Geometry: final body of the model. Coordinates: model frame, mm. A direction names the side the tool comes from. Round coordinates to 2 decimals unless told otherwise and drop trailing zeros. Loops run counter-clockwise (first coordinate to the right, second up) from the corner with the lowest first, then second, coordinate; pieces in that order, holes last. Notation, with made-up numbers: (12.25, 12.25) - (62.25, 12.25) arc R19 cw to (62.25, 25.25) - close; hole circle Ø6 at (73, 14.25). An arc over 180 degrees is marked (long way). Write item = value, one per line. Start each with the question number.
Item 1: Section A-A (y = 33). Return loops of the section in (x, z) (3 decimals).
Item 2: Line query: line 1 (X direction, y = 39, z = 0); line 2 (Y direction, x = -76, z = 5); line 3 (X direction, y = 25, z = 0). Output: solid intervals per line, ascending. Write a range as from..to.
Item 3: First-contact query: pin 1 (8.5 mm diameter, centred on x = 16, y = 30.5, fed in from -Z); pin 2 (4 mm diameter, centred on y = 8, z = -17.5, fed in from -X); pin 3 (10 mm diameter, centred on x = -48.5, y = 12, fed in from +Z); pin 4 (9 mm diameter, centred on x = 0, z = -45, fed in from +Y). Flat tips, straight axial feed; report the tip coordinate or a pass-through.
Item 4: Section C-C (x = 0). Count the separate pieces of the cut face and the enclosed holes in it, plus the area to 4 significant figures.
Item 5: Section D-D (y = 48.5). Return loops of the section in (x, z) (3 decimals), plus the area to 3 significant figures.
Item 6: Section B-B (z = 0). Return loops of the section in (x, y).
Item 7: Access query for faces 4 (the flat face through (0, 37.5, 15)), 5 (the flat face through (67, 15, -1)), 6 (the flat face through (32, 7, 38)), 7 (the flat face through (4, 30, -14)). Directions: +Z, -Z, +X, -X, +Y, -Y. A direction counts if a zero-diameter tool reaches every point of the face in a straight line with its end or side. Return the directions, or none.
Item 8: Draft query along X for faces 1 (the flat face through (-4, 30, 14)), 2 (the cylindrical face through (-87.99, 7.4, -0.83)), 3 (the flat face through (-18, 0, 11)). Return one class per face: pulls with the +X half, pulls with the -X half, needs draft (parallel to the pull), parting line crosses it, or undercut.
from build123d import *

# Parameters (mm, degrees)
SKETCH1_R           = 5
BOSS_EXTRUDE2_DEPTH = 15
CUT_EXTRUDE1_START  = -2
SKETCH2_R           = 10
SKETCH2_R_2         = 5
CUT_EXTRUDE1_DEPTH  = 2
BOSS_EXTRUDE3_START = -15
SKETCH3_R           = 5
BOSS_EXTRUDE3_DEPTH = 25
BOSS_EXTRUDE4_DEPTH = 55
SKETCH5_R           = 27.5
BOSS_EXTRUDE5_DEPTH = 15
SKETCH6_R           = 20
CUT_EXTRUDE2_DEPTH  = 126.175931669
EXTRUDE_THIN1_START = 22.5
EXTRUDE_THIN1_DEPTH = 15
BOSS_EXTRUDE6_START = -15
SKETCH8_R           = 10
BOSS_EXTRUDE6_DEPTH = 20
SKETCH9_R           = 5
CUT_EXTRUDE3_DEPTH  = 113.139483989


with BuildPart() as part:
    # Sketch1 → Boss-Extrude2 (new body)
    with BuildSketch(Plane(origin=(0, 0, 0), x_dir=(1, 0, 0), z_dir=(0, 1, 0))):
        with BuildLine():
            Line((-50.077388597, -38), (50.077388597, -38))
            ThreePointArc((50.077388597, -38), (88.000078802, 0), (50.077388597, 38))
            Line((50.077388597, 38), (-50.077388597, 38))
            ThreePointArc((-50.077388597, 38), (-88.000078802, 0), (-50.077388597, -38))
        make_face()
        with Locations(Location((-60.241162363, 18.755220238, 0), (0, 0, 270))):
            Circle(SKETCH1_R, mode=Mode.SUBTRACT)
        with Locations(Location((-60.241162363, -18.755220238, 0), (0, 0, 270))):
            Circle(SKETCH1_R, mode=Mode.SUBTRACT)
        with Locations(Location((60.241162363, -18.755220238, 0), (0, 0, 270))):
            Circle(SKETCH1_R, mode=Mode.SUBTRACT)
        with Locations(Location((60.241162363, 18.755220238, 0), (0, 0, 270))):
            Circle(SKETCH1_R, mode=Mode.SUBTRACT)
    extrude(amount=BOSS_EXTRUDE2_DEPTH)

    # Sketch2 → Cut-Extrude1 (cut)
    # profile 1 of 4: a face of its own
    with BuildSketch(Plane(origin=(0, 15, 0), x_dir=(1, 0, 0), z_dir=(0, 1, 0)).offset(CUT_EXTRUDE1_START)):
        with Locations(Location((-60.241162363, -18.755220238, 0), (0, 0, 270))):
            Circle(SKETCH2_R)
        with Locations(Location((-60.241162363, -18.755220238, 0), (0, 0, 270))):
            Circle(SKETCH2_R_2, mode=Mode.SUBTRACT)
    # profile 2 of 4: a face of its own
    with BuildSketch(Plane(origin=(0, 15, 0), x_dir=(1, 0, 0), z_dir=(0, 1, 0)).offset(CUT_EXTRUDE1_START)):
        with Locations(Location((-60.241162363, 18.755220238, 0), (0, 0, 270))):
            Circle(SKETCH2_R)
        with Locations(Location((-60.241162363, 18.755220238, 0), (0, 0, 270))):
            Circle(SKETCH2_R_2, mode=Mode.SUBTRACT)
    # profile 3 of 4: a face of its own
    with BuildSketch(Plane(origin=(0, 15, 0), x_dir=(1, 0, 0), z_dir=(0, 1, 0)).offset(CUT_EXTRUDE1_START)):
        with Locations(Location((60.241162363, 18.755220238, 0), (0, 0, 270))):
            Circle(SKETCH2_R)
        with Locations(Location((60.241162363, 18.755220238, 0), (0, 0, 270))):
            Circle(SKETCH2_R_2, mode=Mode.SUBTRACT)
    # profile 4 of 4: a face of its own
    with BuildSketch(Plane(origin=(0, 15, 0), x_dir=(1, 0, 0), z_dir=(0, 1, 0)).offset(CUT_EXTRUDE1_START)):
        with Locations(Location((60.241162363, -18.755220238, 0), (0, 0, 90))):
            Circle(SKETCH2_R)
    extrude(amount=CUT_EXTRUDE1_DEPTH, mode=Mode.SUBTRACT)

    # Sketch3 → Boss-Extrude3 (add)
    with BuildSketch(Plane(origin=(0, 15, 0), x_dir=(1, 0, 0), z_dir=(0, 1, 0)).offset(BOSS_EXTRUDE3_START)):
        with BuildLine():
            Line((-9.21284664, 48.888888889), (-25.33532826, 10.694444444))
            ThreePointArc((-25.33532826, 10.694444444), (-27.5, 0), (-25.33532826, -10.694444444))
            Line((-25.33532826, -10.694444444), (-9.21284664, -48.888888889))
            ThreePointArc((-9.21284664, -48.888888889), (0, -55), (9.21284664, -48.888888889))
            Line((9.21284664, -48.888888889), (25.33532826, -10.694444444))
            ThreePointArc((25.33532826, -10.694444444), (27.5, 0), (25.33532826, 10.694444444))
            Line((25.33532826, 10.694444444), (9.21284664, 48.888888889))
            ThreePointArc((9.21284664, 48.888888889), (0, 55), (-9.21284664, 48.888888889))
        make_face()
        with Locations(Location((0, 45, 0), (0, 0, 270))):
            Circle(SKETCH3_R, mode=Mode.SUBTRACT)
        with Locations(Location((0, -45, 0), (0, 0, 270))):
            Circle(SKETCH3_R, mode=Mode.SUBTRACT)
    extrude(amount=BOSS_EXTRUDE3_DEPTH)

    # Sketch4 → Boss-Extrude4 (add)
    with BuildSketch(Plane(origin=(0, 0, 0), x_dir=(1, 0, 0), z_dir=(0, 1, 0))):
        with BuildLine():
            Line((-53.72, 11.408838679), (-8.525, 26.145255306))
            ThreePointArc((-8.525, 26.145255306), (0, 27.5), (8.525, 26.145255306))
            Line((8.525, 26.145255306), (53.72, 11.408838679))
            ThreePointArc((53.72, 11.408838679), (62, 0), (53.72, -11.408838679))
            Line((53.72, -11.408838679), (8.525, -26.145255306))
            ThreePointArc((8.525, -26.145255306), (0, -27.5), (-8.525, -26.145255306))
            Line((-8.525, -26.145255306), (-53.72, -11.408838679))
            ThreePointArc((-53.72, -11.408838679), (-62, 0), (-53.72, 11.408838679))
        make_face()
    extrude(amount=BOSS_EXTRUDE4_DEPTH)

    # Sketch5 → Boss-Extrude5 (add)
    with BuildSketch(Plane(origin=(0, 55, 0), x_dir=(1, 0, 0), z_dir=(0, 1, 0))):
        with Locations(Location((0, 0, 0), (0, 0, 108.059230491))):
            Circle(SKETCH5_R)
    extrude(amount=BOSS_EXTRUDE5_DEPTH)

    # Sketch6 → Cut-Extrude2 (cut, through all)
    with BuildSketch(Plane(origin=(0, 70, 0), x_dir=(1, 0, 0), z_dir=(0, 1, 0))):
        with Locations(Location((0, 0, 0), (0, 0, 270))):
            Circle(SKETCH6_R)
    extrude(amount=-CUT_EXTRUDE2_DEPTH, mode=Mode.SUBTRACT)

    # Extrude-Thin1: read off the stored shape, not the designer's step
    # Extrude-Thin1 outline → Extrude-Thin1 (add)
    with BuildSketch(Plane(origin=(0, 0, 0), x_dir=(1, 0, 0), z_dir=(0, 1, 0)).offset(EXTRUDE_THIN1_START)):
        with BuildLine():
            Line((4, 4), (4, 19.595917942))
            ThreePointArc((4, 19.595917942), (0, 20), (-4, 19.595917942))
            Line((-4, 19.595917942), (-4, 4))
            Line((-4, 4), (-19.595917942, 4))
            ThreePointArc((-19.595917942, 4), (-20, 0), (-19.595917942, -4))
            Line((-19.595917942, -4), (-4, -4))
            Line((-4, -4), (-4, -19.595917942))
            ThreePointArc((-4, -19.595917942), (0, -20), (4, -19.595917942))
            Line((4, -19.595917942), (4, -4))
            Line((4, -4), (19.595917942, -4))
            ThreePointArc((19.595917942, -4), (20, 0), (19.595917942, 4))
            Line((19.595917942, 4), (4, 4))
        make_face()
    extrude(amount=EXTRUDE_THIN1_DEPTH)

    # Sketch8 → Boss-Extrude6 (add)
    with BuildSketch(Plane(origin=(0, 37.5, 0), x_dir=(1, 0, 0), z_dir=(0, 1, 0)).offset(BOSS_EXTRUDE6_START)):
        with Locations(Location((0, 0, 0), (0, 0, 66.421821522))):
            Circle(SKETCH8_R)
    extrude(amount=BOSS_EXTRUDE6_DEPTH)

    # Sketch9 → Cut-Extrude3 (cut, through all)
    with BuildSketch(Plane(origin=(0, 42.5, 0), x_dir=(1, 0, 0), z_dir=(0, 1, 0))):
        with Locations(Location((0, 0, 0), (0, 0, 270))):
            Circle(SKETCH9_R)
    extrude(amount=-CUT_EXTRUDE3_DEPTH, mode=Mode.SUBTRACT)


solid = part.part
Taken from the geometry:
q1.outline = (-53.72, -11.409) - (-8.525, -26.145) arc R27.5 ccw to (8.525, -26.145) - (53.72, -11.409) arc R12 ccw to (53.72, 11.409) - (8.525, 26.145) arc R27.5 ccw to (-8.525, 26.145) - (-53.72, 11.409) arc R12 ccw to start; hole (-19.596, -4) arc R20 ccw to (-4, -19.596) - (-4, -9.165) arc R10 cw to (-9.165, -4) - close; hole (-19.596, 4) - (-9.165, 4) arc R10 cw to (-4, 9.165) - (-4, 19.596) arc R20 ccw to start; hole circle Ø10 at (0, 0); hole (4, -19.596) arc R20 ccw to (19.596, -4) - (9.165, -4) arc R10 cw to (4, -9.165) - close; hole (4, 9.165) arc R10 cw to (9.165, 4) - (19.596, 4) arc R20 ccw to (4, 19.596) - close
q2.line_1 = -62..-20, -10..-5, 5..10, 20..62
q2.line_2 = 0..15
q2.line_3 = -62..-5, 5..62
q3.pin_1 = -25.09
q3.pin_2 = -84.7
q3.pin_3 = 38
q3.pin_4 = through
q4.separate_pieces = 4
q4.enclosed_holes = 0
q4.area = 2,425 mm^2
q5.outline = (-53.72, -11.409) - (-8.525, -26.145) arc R27.5 ccw to (8.525, -26.145) - (53.72, -11.409) arc R12 ccw to (53.72, 11.409) - (8.525, 26.145) arc R27.5 ccw to (-8.525, 26.145) - (-53.72, 11.409) arc R12 ccw to start; hole circle Ø40 at (0, 0)
q5.area = 3,340 mm^2
q6.outline = (-88, 0) - (-20, 0) - (-20, 22.5) - (-5, 22.5) - (-5, 42.5) - (-10, 42.5) - (-10, 37.5) - (-20, 37.5) - (-20, 70) - (-27.5, 70) - (-27.5, 55) - (-62, 55) - (-62, 15) - (-88, 15) - close; (5, 22.5) - (20, 22.5) - (20, 0) - (88, 0) - (88, 15) - (62, 15) - (62, 55) - (27.5, 55) - (27.5, 70) - (20, 70) - (20, 37.5) - (10, 37.5) - (10, 42.5) - (5, 42.5) - close
q7.face_4 = +Y
q7.face_5 = +X, +Y
q7.face_6 = +Z, +X, +Y, -Y
q7.face_7 = +Y, -Y
q8.face_1 = undercut
q8.face_2 = pulls with the -X half
q8.face_3 = needs draft
